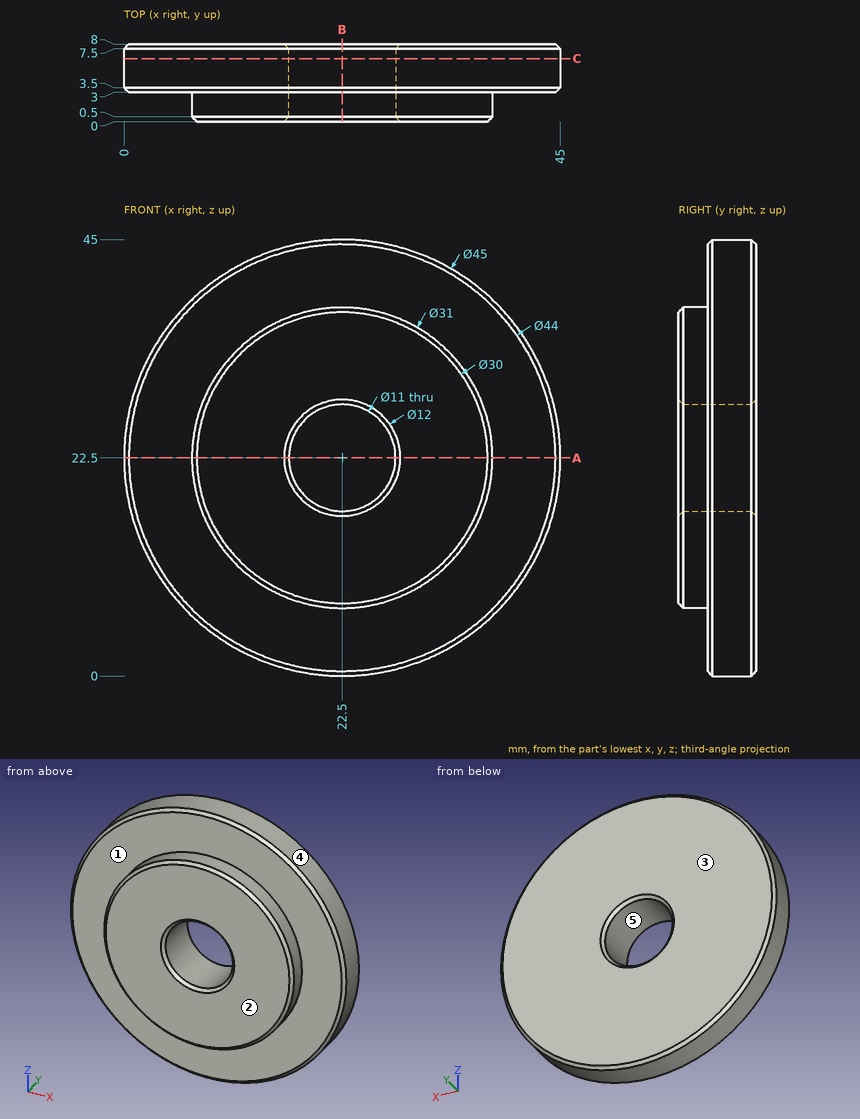
Study the drawing (mm; zero at the part's minimum x, y, z) and answer. A direction names the side the tool comes from. Give positions to 0.01 mm unless a question says otherwise; leave off trailing zeros. Write each loop counter-clockwise with the first axis right and the second up, starting at its lowest first coordinate (ties: lowest second). Pieces come first, ordered by that corner, then holes. Notation, with made-up numbers: (60.5, -27.5) - (82.5, -27.5) arc R32 ccw to (82.5, 7.5) - close; hole circle Ø3 at (-21, -13). An arc over 180 degrees is marked (long way). Write item = value, one per line. Start each with the question number.
Item 1: Find section B-B (x = 22.5). Give the vertices of the cut face in (y, z).
Item 2: Each of these flat-tipped pins is pushed along its axis until it touches: P1, Ø6, axis at x = 33, z = 39, coming from the -Y side; P2, Ø1, axis at y = 4, z = 28.5, coming from the -X side. Where does it stop, or does it pass through?
Item 3: Find section A-A (z = 22.5). Give the vertices of the cut face in (x, y).
Item 4: Find section C-C (y = 6.5). Give the vertices of the cut face in (x, z), then the cut area to 3 significant figures.
Item 5: Find the intervals of material crossed by probe 1 along Z at (x, y) = (22.5, 3.5); probe 2 along Z at (x, y) = (22.5, 2.25); probe 3 along X at (y, z) = (6.5, 18.5), in increasing order. Write a range as [from, to].
Item 6: The mould has two halves that part along X. Classify the marked faces 3, 4 and 5: +X half, -X half, draft (parallel to the pull), parting line (faces both ways), or undercut.
Item 7: A tool of negligible diameter and unlimited length cuts with its end or side. For the marked faces 1 and 2, from which of +Z, -Z, +X, -X, +Y, -Y can it reach the whole face along a straight path? Write none if from no direction.
Response:
q1.outline = (0, 7.5) - (0.5, 7) - (3, 7) - (3, 0.5) - (3.5, 0) - (7.5, 0) - (8, 0.5) - (8, 16.5) - (7.5, 17) - (0.5, 17) - (0, 16.5) - close; (0, 28.5) - (0.5, 28) - (7.5, 28) - (8, 28.5) - (8, 44.5) - (7.5, 45) - (3.5, 45) - (3, 44.5) - (3, 38) - (0.5, 38) - (0, 37.5) - close
q2.P1 = 3
q2.P2 = 0.68
q3.outline = (0, 3.5) - (0.5, 3) - (7, 3) - (7, 0.5) - (7.5, 0) - (16.5, 0) - (17, 0.5) - (17, 7.5) - (16.5, 8) - (0.5, 8) - (0, 7.5) - close; (28, 0.5) - (28.5, 0) - (37.5, 0) - (38, 0.5) - (38, 3) - (44.5, 3) - (45, 3.5) - (45, 7.5) - (44.5, 8) - (28.5, 8) - (28, 7.5) - close
q4.outline = circle Ø45 at (22.5, 22.5); hole circle Ø11 at (22.5, 22.5)
q4.area = 1,500 mm²
q5.probe_1 = [0, 17], [28, 45]
q5.probe_2 = [7, 17], [28, 38]
q5.probe_3 = [0.36, 18.73], [26.27, 44.64]
q6.face_3 = draft
q6.face_4 = parting line
q6.face_5 = undercut
q7.face_1 = -Y
q7.face_2 = +Z, -Z, +X, -X, -Y
